Work out the finished part from the listing and answer in its coordinate system (mm). Round coordinates to 2 decimals unless told otherwise and drop trailing zeros. Loops run counter-clockwise (first coordinate to the right, second up) from the corner with the lowest first, then second, coordinate; pieces in that order, holes last. Notation, with made-up numbers: (0, 1) - (23, 1) arc R22 ccw to (23, 10) - close; hole circle Ø10 at (83, 48). An arc over 180 degrees is marked (long way). Use CSV: the item, a comma, the result in double quotes. Start each with the question number.
from build123d import *

# Parameters (mm, degrees)
SKETCH1_W           = 457.2
SKETCH1_H           = 76.2
BOSS_EXTRUDE1_DEPTH = 12.7
CUT_EXTRUDE1_DEPTH  = 12.7
SKETCH3_R           = 15.5575
CUT_EXTRUDE2_DEPTH  = 12.7


with BuildPart() as part:
    # Sketch1 → Boss-Extrude1 (new body)
    with BuildSketch(Plane.XY):
        with Locations((228.6, 38.1)):
            Rectangle(SKETCH1_W, SKETCH1_H)
    extrude(amount=BOSS_EXTRUDE1_DEPTH)

    # Sketch2 → Cut-Extrude1 (cut)
    with BuildSketch(Plane.XY.offset(12.7)):
        Polygon((0, 0), (117.088214608, 76.2), (0, 76.2), align=None)
    extrude(amount=-CUT_EXTRUDE1_DEPTH, mode=Mode.SUBTRACT)

    # Sketch3 → Cut-Extrude2 (cut)
    with BuildSketch(Plane.XY.offset(12.7)):
        with Locations((63.5, 19.05)):
            Circle(SKETCH3_R)
        with Locations((431.8, 38.1)):
            Circle(SKETCH3_R)
    extrude(amount=-CUT_EXTRUDE2_DEPTH, mode=Mode.SUBTRACT)


solid = part.part
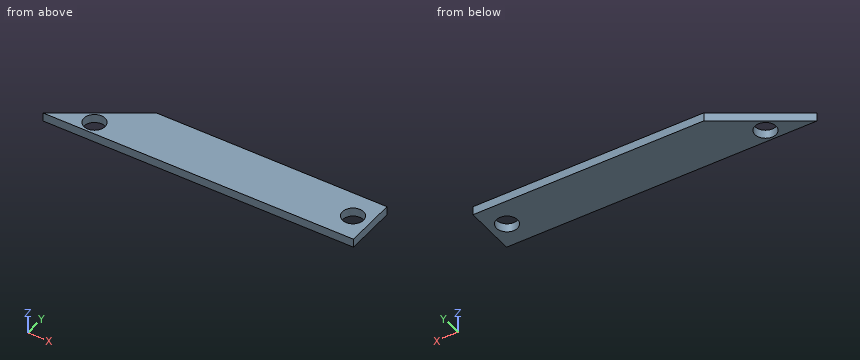
Item 1: Find the intervals of material crossed by probe 1 along X at (y, z) = (26, 4.75); probe 2 along Y at (x, z) = (431.8, 5); probe 3 along X at (y, z) = (33.5, 2), in increasing order. Write a range as [from, to].
Item 2: A cutting plane is placed at C-C (z = 3.25). State how many separate pieces and enclosed holes the cut face has, plus the area to 3 significant figures.
Item 3: A cutting plane is placed at B-B (y = 8.5). Determine the outline of the cut face in (x, z), plus the area to 3 significant figures.
Item 4: A cutting plane is placed at D-D (y = 64). Determine the outline of the cut face in (x, z), plus the area to 3 significant figures.
Item 5: A cutting plane is placed at A-A (x = 431.8). Determine the outline of the cut face in (y, z), plus the area to 3 significant figures.
Result sheet:
1,probe 1,"[39.95, 49.58], [77.42, 422.02], [441.58, 457.2]"
1,probe 2,"[0, 22.54], [53.66, 76.2]"
1,probe 3,"[51.48, 57.74], [69.26, 416.94], [446.66, 457.2]"
2,separate pieces,"1"
2,enclosed holes,"2"
2,area,"28,900 mm^2"
3,outline,"(13.06, 0) - (52.07, 0) - (52.07, 12.7) - (13.06, 12.7) - close; (74.93, 0) - (457.2, 0) - (457.2, 12.7) - (74.93, 12.7) - close"
3,area,"5,350 mm^2"
4,outline,"(98.34, 0) - (457.2, 0) - (457.2, 12.7) - (98.34, 12.7) - close"
4,area,"4,560 mm^2"
5,outline,"(0, 0) - (22.54, 0) - (22.54, 12.7) - (0, 12.7) - close; (53.66, 0) - (76.2, 0) - (76.2, 12.7) - (53.66, 12.7) - close"
5,area,"573 mm^2"
